Build history of the part. All positions in model axes, mm. Face numbers are marked on the shaded views. A direction names the side the tool comes from. Round coordinates to 2 decimals unless told otherwise and drop trailing zeros. Write each loop counter-clockwise with the first axis right and the second up, starting at its lowest first coordinate (ties: lowest second). Pieces come first, ordered by that corner, then holes. Notation, with made-up numbers: (-39, -16.5) -> (-1, -16.5) arc R33 ccw to (-1, 15.5) -> close; hole circle Ø9 at (89, -26). An arc over 180 degrees is marked (long way). Return JSON: item names as keys, results as strings.
from build123d import *

# Parameters (mm, degrees)
SKETCH1_W           = 16.6624
SKETCH1_H           = 37.2872
BOSS_EXTRUDE1_DEPTH = 100
BOSS_EXTRUDE2_DEPTH = 18.6436
SKETCH2_3_W         = 8.2312
SKETCH2_3_H         = 29.9
SKETCH2_3_H_2       = 0.1
BOSS_EXTRUDE3_DEPTH = 15
SKETCH3_R           = 3.2
CUT_EXTRUDE1_DEPTH  = 151.542823877
FILLET1_R           = 6
FILLET3_R           = 2.2
FILLET2_R           = 0.5
FILLET4_R           = 1
CHAMFER1_SIZE       = 0.4


with BuildPart() as part:
    # Sketch1 → Boss-Extrude1 (new, symmetric)
    with BuildSketch(Plane(origin=(0, 0, 0), x_dir=(0, 1, 0), z_dir=(0, 0, 1))):
        Rectangle(SKETCH1_W, SKETCH1_H)
    extrude(amount=BOSS_EXTRUDE1_DEPTH, both=True)


with BuildPart() as body_2:
    # Sketch2 → Boss-Extrude2 (new body)
    with BuildSketch(Plane.YZ.offset(18.6436)):
        Polygon((-8.3312, -100), (-8.3312, -70.1), (-19.1, -70.1), (-19.1, -145.5), (-0.1, -145.5), (-0.1, -130.5), (-15.2, -130.5), (-15.2, -100.1), (-8.3312, -100.1), align=None)
    extrude(amount=-BOSS_EXTRUDE2_DEPTH)

    # Sketch2<3> → Boss-Extrude3 (add)
    with BuildSketch(Plane.YZ.offset(18.6436)):
        Polygon((-8.3312, -100), (-8.3312, -70.1), (-19.1, -70.1), (-19.1, -145.5), (-0.1, -145.5), (-0.1, -130.5), (-15.2, -130.5), (-15.2, -100.1), (-8.3312, -100.1), align=None)
        with Locations((-4.2156, -85.05)):
            Rectangle(SKETCH2_3_W, SKETCH2_3_H)
        with Locations((-4.2156, -100.05)):
            Rectangle(SKETCH2_3_W, SKETCH2_3_H_2)
    extrude(amount=BOSS_EXTRUDE3_DEPTH)

    # Sketch3 → Cut-Extrude1 (cut, through all)
    with BuildSketch(Plane.XZ.offset(19.1)):
        Polygon((15.46262002, -134.5), (0, -134.5), (0, -145.5), (21.813472981, -145.5), align=None)
        with Locations(Location((26.1436, -138, 0), (0, 0, 270))):
            Circle(SKETCH3_R)
        with Locations(Location((26.1436, -90.206601718, 0), (0, 0, 270))):
            Circle(SKETCH3_R)
        Polygon((33.6436, -70.1), (18.6436, -70.1), (18.6436, -72.1), (33.6436, -87.1), align=None)
        Polygon((18.6436, -70.1), (16.6436, -70.1), (18.6436, -72.1), align=None)
        with Locations(Location((9.3218, -77.6, 0), (0, 0, 270))):
            Circle(SKETCH3_R)
        with Locations(Location((9.3218, -92.6, 0), (0, 0, 270))):
            Circle(SKETCH3_R)
    extrude(amount=-CUT_EXTRUDE1_DEPTH, mode=Mode.SUBTRACT)

    # Fillet1
    fillet1_edges = [body_2.edges().sort_by_distance(p)[0] for p in [
        (15.46262002, -9.6, -134.5),
        (21.813472981, -9.6, -145.5),
        (33.6436, -9.6, -145.5),
        (16.6436, -13.7156, -70.1),
        (33.6436, -9.6, -87.1),
    ]]
    fillet(fillet1_edges, radius=FILLET1_R)

    # Fillet3
    fillet3_edges = [body_2.edges().sort_by_distance(p)[0] for p in [
        (16.8218, -15.2, -130.5),
        (16.8218, -15.2, -100.1),
    ]]
    fillet(fillet3_edges, radius=FILLET3_R)

    # Fillet2
    fillet2_edges = [body_2.edges().sort_by_distance(p)[0] for p in [
        (33.6436, -6.55, -130.5),
        (33.6436, -15.2, -115.3),
        (33.6436, -14.555634919, -129.855634919),
        (33.6436, -14.555634919, -100.744365081),
        (33.6436, -6.55, -100.1),
        (18.6436, -4.2156, -100.1),
    ]]
    fillet(fillet2_edges, radius=FILLET2_R)

    # Fillet4
    fillet4_edges = [body_2.edges().sort_by_distance(p)[0] for p in [
        (18.6436, -4.2156, -72.1),
    ]]
    fillet(fillet4_edges, radius=FILLET4_R)

    # Chamfer1
    chamfer1_edges = [body_2.edges().sort_by_distance(p)[0] for p in [
        (26.1436, -0.1, -87.006601718),
        (26.1436, -19.1, -87.006601718),
        (26.1436, -0.1, -134.8),
        (26.1436, -19.1, -134.8),
        (9.3218, -8.3312, -89.4),
        (9.3218, -19.1, -89.4),
        (5.999259202, -19.1, -134.5),
        (5.999259202, -0.1, -134.5),
        (26.460587298, -0.1, -145.5),
        (26.460587298, -19.1, -145.5),
        (33.6436, -19.1, -114.542640687),
        (25.1436, -19.1, -78.6),
        (18.638046501, -19.1, -140),
        (16.45441922, -19.1, -70.556722805),
        (33.186877195, -19.1, -87.28918078),
        (22.277574596, -19.1, -144.696152423),
        (31.886240687, -19.1, -143.742640687),
        (18.638046501, -0.1, -140),
        (22.277574596, -0.1, -144.696152423),
        (31.886240687, -0.1, -143.742640687),
        (19.375833047, -8.3312, -72.832233047),
        (33.186877195, -0.1, -87.28918078),
        (16.45441922, -8.3312, -70.556722805),
        (14.998518405, -19.1, -135.303847577),
        (14.998518405, -0.1, -135.303847577),
        (33.6436, -0.1, -135.25),
        (33.6436, -0.1, -94.592640687),
        (33.497153391, -0.1, -130.646446609),
        (18.6436, -0.1, -87.057106781),
        (26.1436, -0.1, -100.1),
        (33.497153391, -0.1, -99.953553391),
        (18.790046609, -0.1, -99.953553391),
        (26.118473734, -0.1, -79.574873734),
        (19.260916568, -0.1, -73.59033403),
        (7.079159313, -19.1, -70.1),
        (16.5718, -0.1, -130.5),
        (9.5718, -8.3312, -100.1),
        (7.079159313, -8.3312, -70.1),
        (9.3218, -8.3312, -74.4),
        (9.3218, -19.1, -74.4),
    ]]
    chamfer(chamfer1_edges, length=CHAMFER1_SIZE)

    # Mirror1: body 2 across plane


with BuildPart() as body_2_1:
    add(body_2.part)
    add(body_2.part.mirror(Plane(origin=(0, 0, 0), x_dir=(0, 0, 1), z_dir=(1, 0, 0))))


solid = body_2_1.part
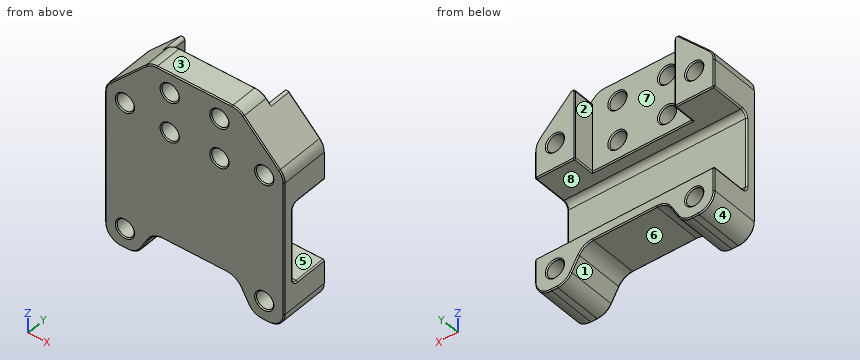
Q1. Two-plate mould, pull along Z, no slides. Class the marked faces 6, 7 and 8: +Z half, -Z half, draft (parallel to the pull), parting line (faces both ways), or undercut.
Verdict:
{"face 6": "-Z half", "face 7": "draft", "face 8": "undercut"}
Q2. Saw through at A-A on z = -77.6. Count the separate pieces of the cut face and the enclosed holes in it, then the cut area to 3 significant figures.
Verdict:
{"separate pieces": "3", "enclosed holes": "0", "area": "471 mm²"}
Q3. Pin check, flat tips, straight feed: pin 1 Ø8 at (x, z) = (-13.5, -116.5) entering from +Y; pin 2 Ø10 at (x, y) = (-2.5, -3.5) entering from -Z; pin 3 Ø1.5 at (y, z) = (-11.5, -84.5) entering from -X; pin 4 Ø5 at (x, z) = (26.14, -138) entering from +Y. Stop position of each tip, or through.
Verdict:
{"pin 1": "stops at y = -15.2", "pin 2": "stops at z = -134.5", "pin 3": "stops at x = -31.79", "pin 4": "passes through"}
Q4. Saw through at B-B on z = -116. List the corners of the cut face in (x, y), then the cut area to 3 significant figures.
Verdict:
{"outline": "(-33.64, -18.7) -> (-33.24, -19.1) -> (33.24, -19.1) -> (33.64, -18.7) -> (33.64, -15.7) arc R0.5 ccw to (33.14, -15.2) -> (-33.14, -15.2) arc R0.5 ccw to (-33.64, -15.7) -> close", "area": "262 mm²"}
Q5. 3-axis set-ups, long thin cutter, end or side, ignore diameter. For the marked faces 1, 2, 3, 4 and 5: which of +Z, -Z, +X, -X, +Y, -Y reach the whole face in a straight line?
Verdict:
{"face 1": "-Z, +Y, -Y", "face 2": "+Z, +Y", "face 3": "+Z, +X, -X, +Y, -Y", "face 4": "-Z, -X, +Y, -Y", "face 5": "+X, -X, +Y"}
Q6. Wall check: L1, parallel to Z at x = -5, y = -13; L2, parallel to X at y = -12.75, z = -138; L3, parallel to Z at x = 27, y = -11.75. Give the ranges that are in metal, low to high.
Verdict:
{"L1": "z = -134.5 to -130.5, -100.1 to -70.1", "L2": "x = -33.64 to -29.34, -22.94 to -17.48, 17.48 to 22.94, 29.34 to 33.64", "L3": "z = -145.5 to -141.08, -134.92 to -130.5, -100.1 to -93.29, -87.12 to -80.46"}
